```python
from build123d import *

# Parameters (mm, degrees)
BOSS_EXTRUDE1_DEPTH                            = 76.2
F_18_0MM_DIAMETER_HOLE1_D                      = 18
CBORE_FOR_M5_HEX_HEAD_BOLT1_D                  = 5.5
CBORE_FOR_M5_HEX_HEAD_BOLT1_DEPTH              = 45.974
CBORE_FOR_M5_HEX_HEAD_BOLT1_CBORE_D            = 12.24
CBORE_FOR_M5_HEX_HEAD_BOLT1_CBORE_DEPTH        = 3.58
CBORE_FOR_M5_HEX_HEAD_BOLT1_TIP                = 1.652366702
CBORE_FOR_4_SOCKET_HEAD_CAP_SCREW1_D           = 3.2639
CBORE_FOR_4_SOCKET_HEAD_CAP_SCREW1_DEPTH       = 45.974
CBORE_FOR_4_SOCKET_HEAD_CAP_SCREW1_CBORE_D     = 5.55752
CBORE_FOR_4_SOCKET_HEAD_CAP_SCREW1_CBORE_DEPTH = 2.8448
CBORE_FOR_4_SOCKET_HEAD_CAP_SCREW1_TIP         = 0.980574487
F_10_CLEARANCE_HOLE1_D                         = 5.1054
CUT_EXTRUDE2_DEPTH                             = 26.4
CUT_EXTRUDE2_DEPTH_BACK                        = 1
CBORE_FOR_1_4_HEX_MACHINE_SCREW1_D             = 6.7564
CBORE_FOR_1_4_HEX_MACHINE_SCREW1_CBORE_D       = 15.875
CBORE_FOR_1_4_HEX_MACHINE_SCREW1_CBORE_DEPTH   = 4.826


with BuildPart() as part:
    # Sketch1 → Boss-Extrude1 (new body)
    with BuildSketch(Plane.XY):
        Polygon((0, 0), (0, 9.525), (17.4625, 9.525), (17.4625, 79.375), (25.4, 79.375), (25.4, 0), align=None)
    extrude(amount=BOSS_EXTRUDE1_DEPTH)

    # Ø18.0mm Diameter Hole1 (through all)
    with Locations(Plane(origin=(25.4, 0, 0), x_dir=(0, 0, -1), z_dir=(1, 0, 0))):
        with Locations((-47.625, 42.8625)):
            Hole(F_18_0MM_DIAMETER_HOLE1_D / 2)

    # CBORE for M5 Hex Head Bolt1
    with Locations(Plane.ZY.offset(-17.4625)):
        with Locations((49.803893572, 67.76736749), (45.446106428, 17.95763251)):
            CounterBoreHole(CBORE_FOR_M5_HEX_HEAD_BOLT1_D / 2, CBORE_FOR_M5_HEX_HEAD_BOLT1_CBORE_D / 2, CBORE_FOR_M5_HEX_HEAD_BOLT1_CBORE_DEPTH, depth=CBORE_FOR_M5_HEX_HEAD_BOLT1_DEPTH)
            with Locations((0, 0, -(CBORE_FOR_M5_HEX_HEAD_BOLT1_DEPTH + CBORE_FOR_M5_HEX_HEAD_BOLT1_TIP / 2))):  # 118° drill point
                Cone(0, CBORE_FOR_M5_HEX_HEAD_BOLT1_D / 2, CBORE_FOR_M5_HEX_HEAD_BOLT1_TIP, mode=Mode.SUBTRACT)

    # CBORE for #4 Socket Head Cap Screw1
    with Locations(Plane(origin=(25.4, 0, 0), x_dir=(0, 0, -1), z_dir=(1, 0, 0))):
        with Locations((-24.453273137, 57.320623121), (-63.5, 65.0875)):
            CounterBoreHole(CBORE_FOR_4_SOCKET_HEAD_CAP_SCREW1_D / 2, CBORE_FOR_4_SOCKET_HEAD_CAP_SCREW1_CBORE_D / 2, CBORE_FOR_4_SOCKET_HEAD_CAP_SCREW1_CBORE_DEPTH, depth=CBORE_FOR_4_SOCKET_HEAD_CAP_SCREW1_DEPTH)
            with Locations((0, 0, -(CBORE_FOR_4_SOCKET_HEAD_CAP_SCREW1_DEPTH + CBORE_FOR_4_SOCKET_HEAD_CAP_SCREW1_TIP / 2))):  # 118° drill point
                Cone(0, CBORE_FOR_4_SOCKET_HEAD_CAP_SCREW1_D / 2, CBORE_FOR_4_SOCKET_HEAD_CAP_SCREW1_TIP, mode=Mode.SUBTRACT)

    # #10 Clearance Hole1 (through all)
    with Locations(Plane.ZY.offset(-17.4625)):
        with Locations((6.35, 24.863549414), (12.7, 24.863549414), (6.35, 19.395959874), (12.7, 19.395959874)):
            Hole(F_10_CLEARANCE_HOLE1_D / 2)

    # Sketch10 → Cut-Extrude2 (cut, two sides)
    with BuildSketch(Plane(origin=(0, 0, 0), x_dir=(0, 0, -1), z_dir=(1, 0, 0))) as cut_extrude2_sk:
        with BuildLine():
            ThreePointArc((-74.909422182, 25.327542498), (-75.876819337, 17.452577507), (-76.2, 9.525))
            Line((-76.2, 9.525), (-76.2, 79.375))
            Line((-76.2, 79.375), (0, 79.375))
            Line((0, 79.375), (0, 9.525))
            ThreePointArc((0, 9.525), (-0.160347065, 17.432771339), (-0.641124655, 25.327542498))
            ThreePointArc((-0.641124655, 25.327542498), (-0.890670545, 26.596255157), (-1.418437728, 27.776664731))
            Line((-1.418437728, 27.776664731), (-20.314478636, 59.765443848))
            ThreePointArc((-20.314478636, 59.765443848), (-21.017481453, 60.682483292), (-21.919014013, 61.405264965))
            Line((-21.919014013, 61.405264965), (-44.903501732, 75.665670144))
            ThreePointArc((-44.903501732, 75.665670144), (-49.642737782, 77.060970334), (-54.427500457, 75.830821116))
            Line((-54.427500457, 75.830821116), (-65.891118571, 69.257550393))
            ThreePointArc((-65.891118571, 69.257550393), (-67.449429859, 67.827713877), (-68.243251822, 65.867455417))
            Line((-68.243251822, 65.867455417), (-74.909422182, 25.327542498))
        make_face()
    extrude(amount=CUT_EXTRUDE2_DEPTH, mode=Mode.SUBTRACT)
    extrude(cut_extrude2_sk.sketch, amount=-CUT_EXTRUDE2_DEPTH_BACK, mode=Mode.SUBTRACT)

    # CBORE for 1/4 Hex Machine Screw1 (through all)
    with Locations(Plane(origin=(0, 9.525, 0), x_dir=(1, 0, 0), z_dir=(0, 1, 0))):
        with Locations((8.73125, -19.05), (8.73125, -57.15)):
            CounterBoreHole(CBORE_FOR_1_4_HEX_MACHINE_SCREW1_D / 2, CBORE_FOR_1_4_HEX_MACHINE_SCREW1_CBORE_D / 2, CBORE_FOR_1_4_HEX_MACHINE_SCREW1_CBORE_DEPTH)


solid = part.part
```
Source: CAD feature listing. Evaluate the final solid. Frame: model axes, mm. A direction names the side the tool comes from. Coordinates: 2 decimals unless noted, no trailing zeros. Order: outer loops, then holes, each group sorted by start corner. A loop starts at its lowest first (then second) coordinate and runs counter-clockwise, first axis right, second up. Notation, with made-up numbers: (74, 35.25) - (115, 35.25) arc R21 cw to (115, 59.25) - close; hole circle Ø9 at (2.5, -38). An arc over 180 degrees is marked (long way). One line per item, written item: value.
1) Cut plane B-B on x = 7. Output: boundary loops of the cut face in (y, z) (3 decimals).
Computed values:
outline: (0, 0) - (9.525, 0) - (9.525, 11.304) - (4.699, 11.304) - (4.699, 16.149) - (0, 16.149) - close; (0, 21.951) - (4.699, 21.951) - (4.699, 26.796) - (9.525, 26.796) - (9.525, 49.404) - (4.699, 49.404) - (4.699, 54.249) - (0, 54.249) - close; (0, 60.051) - (4.699, 60.051) - (4.699, 64.896) - (9.525, 64.896) - (9.525, 76.2) - (0, 76.2) - close
2) Cut plane A-A on z = 12.7. State how many separate pieces and enclosed holes the cut face has, plus the area to 3 significant figures.
Computed values:
separate pieces: 3
enclosed holes: 0
area: 411 mm^2
3) Mould query, pull axis X, two halves, no side actions, for faces 5 (the face through (21.042, 65, 51)), 6 (the face through (9.17, 2.32, 15.7)), 7 (the face through (21.376, 34.077, 45.674)). Classes: released by +X, released by -X, zero draft, split by the parting line, or undercut.
Computed values:
face 5: released by -X
face 6: undercut
face 7: zero draft
4) Reachability of faces 1 (the face through (12.394, 7.146, 26.092)), 2 (the face through (13, 5, 0)), 3 (the face through (23.998, 60.076, 24.815)), 4 (the face through (19.227, 19.796, 51.283)) from +Z, -Z, +X, -X, +Y, -Y: full face, straight path, thin tool, end or side. Return the list, or none.
Computed values:
face 1: +Y
face 2: -Z, +X, -X, +Y, -Y
face 3: +X
face 4: -X
5) Cut plane C-C on z = 63.5. Output: boundary loops of the cut face in (x, y) (1 decimal), plus the area to 3 significant figures.
Computed values:
outline: (0, 0) - (25.4, 0) - (25.4, 62.3) - (22.6, 62.3) - (22.6, 63.5) - (17.5, 63.5) - (17.5, 9.5) - (13.5, 9.5) - (13.5, 4.7) - (4, 4.7) - (4, 9.5) - (0, 9.5) - close; (17.5, 66.7) - (22.6, 66.7) - (22.6, 67.9) - (25.4, 67.9) - (25.4, 70.6) - (17.5, 70.6) - close
area: 649 mm^2
6) Contact query for flat-ended pins moving along their axis: pin 1 (12.5 mm diameter, centred on x = 8, z = 22, fed in from +Y) (3 decimals); pin 2 (8 mm diameter, centred on x = 19.5, y = 36.5, fed in from -Z); pin 3 (8 mm diameter, centred on x = 14.5, y = 17.5, fed in from -Z). Output: stop coordinate, or through.
Computed values:
pin 1: stops at y = 9.525
pin 2: stops at z = 4.21
pin 3: stops at z = 0.07
7) Ray query, line 1 (Y direction, x = 20.5, z = 11.5); line 2 (Y direction, x = 22.25, z = 12.7); line 3 (X direction, y = 11.5, z = 21.5). Return the intervals inside material, ascending. Write a range as [from, to].
Computed values:
line 1: y = [0, 17.14], [21.65, 22.61], [27.12, 44.84]
line 2: y = [0, 16.84], [21.95, 22.31], [27.42, 46.88]
line 3: x = [17.46, 25.4]
8) Cut plane D-D on y = 31. Output: boundary loops of the cut face in (x, z).
Computed values:
outline: (17.46, 3.32) - (25.4, 3.32) - (25.4, 73.98) - (17.46, 73.98) - close
